from build123d import *

# Parameters (mm, degrees)
F0_R     = 100
F0_R_2   = 9
F0_R_3   = 50
F0_R_4   = 40
F1_DEPTH = 20
F2_DEPTH = 500
F3_R     = 100
F3_R_2   = 9
F3_R_3   = 50
F3_R_4   = 40
F4_DEPTH = 20


with BuildPart() as f1:
    # F0 (on Front) → F1 (new body)
    with BuildSketch(Plane.XZ):
        Circle(F0_R)
        with Locations((-56.5685424949, -56.5685424949)):
            Circle(F0_R_2, mode=Mode.SUBTRACT)
        with Locations((0, -80)):
            Circle(F0_R_2, mode=Mode.SUBTRACT)
        with Locations((56.5685424949, -56.5685424949)):
            Circle(F0_R_2, mode=Mode.SUBTRACT)
        with Locations((-80, 0)):
            Circle(F0_R_2, mode=Mode.SUBTRACT)
        with Locations((-56.5685424949, 56.5685424949)):
            Circle(F0_R_2, mode=Mode.SUBTRACT)
        Circle(F0_R_3, mode=Mode.SUBTRACT)
        with Locations((80, 0)):
            Circle(F0_R_2, mode=Mode.SUBTRACT)
        with Locations((0, 80)):
            Circle(F0_R_2, mode=Mode.SUBTRACT)
        with Locations((56.5685424949, 56.5685424949)):
            Circle(F0_R_2, mode=Mode.SUBTRACT)
        Circle(F0_R_3)
        Circle(F0_R_4, mode=Mode.SUBTRACT)
    extrude(amount=F1_DEPTH)

    # F0 (on Front) → F2 (join)
    with BuildSketch(Plane.XZ):
        Circle(F0_R_3)
        Circle(F0_R_4, mode=Mode.SUBTRACT)
    extrude(amount=F2_DEPTH)

    # F3 (on face) → F4 (join)
    with BuildSketch(Plane.XZ.offset(500)):
        Circle(F3_R)
        with Locations((-56.5685424949, -56.5685424949)):
            Circle(F3_R_2, mode=Mode.SUBTRACT)
        with Locations((0, -80)):
            Circle(F3_R_2, mode=Mode.SUBTRACT)
        with Locations((56.5685424949, -56.5685424949)):
            Circle(F3_R_2, mode=Mode.SUBTRACT)
        with Locations((-80, 0)):
            Circle(F3_R_2, mode=Mode.SUBTRACT)
        with Locations((-56.5685424949, 56.5685424949)):
            Circle(F3_R_2, mode=Mode.SUBTRACT)
        Circle(F3_R_3, mode=Mode.SUBTRACT)
        with Locations((80, 0)):
            Circle(F3_R_2, mode=Mode.SUBTRACT)
        with Locations((0, 80)):
            Circle(F3_R_2, mode=Mode.SUBTRACT)
        with Locations((56.5685424949, 56.5685424949)):
            Circle(F3_R_2, mode=Mode.SUBTRACT)
        Circle(F3_R_3)
        Circle(F3_R_4, mode=Mode.SUBTRACT)
    extrude(amount=F4_DEPTH)


solid = f1.part
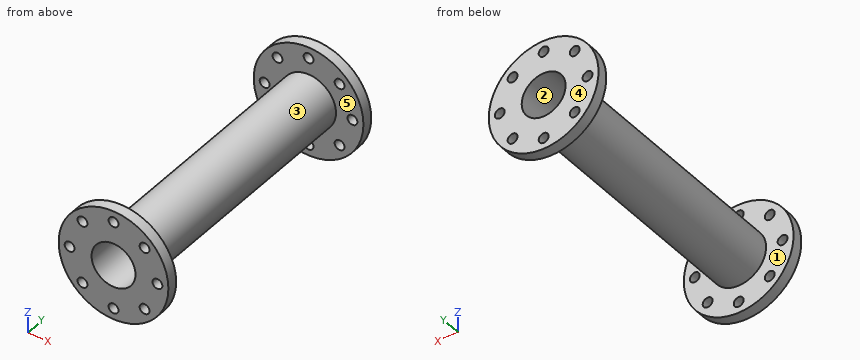
The model under review builds one solid part; all positions refer to its coordinate system, in mm. Face numbers are marked on the shaded views. A direction names the side the tool comes from. Coordinates: 2 decimals unless noted, no trailing zeros. Write each loop counter-clockwise with the first axis right and the second up, starting at its lowest first coordinate (ties: lowest second). Pieces come first, ordered by that corner, then holes. Notation, with made-up numbers: (51.25, 59.25) - (68.25, 59.25) arc R29 cw to (68.25, 91.25) - close; hole circle Ø6 at (2.5, 81). An arc over 180 degrees is marked (long way). Answer as CSV lines item,"result".
(1) Mouldability with a two-part tool opening along X and no side actions: class the marked faces 1, 2 and 3 as pulls with the +X half, pulls with the -X half, needs draft (parallel to the pull), parting line crosses it, or undercut.
Data:
face 1,"needs draft"
face 2,"undercut"
face 3,"parting line crosses it"
(2) For line 1 along Y through (x, z) = (-75, 43); line 2 along Z through (x, y) = (0, -13.5); line 3 along Z through (x, y) = (80, -5.25), list the stretches that pass through material, from the lowest coordinate up. Write a range as [from, to].
Data:
line 1,"y = [-520, -500], [-20, 0]"
line 2,"z = [-100, -89], [-71, -40], [40, 71], [89, 100]"
line 3,"z = [-60, -9], [9, 60]"
(3) We need section B-B (z = -80). Give the boundary of the cut face in (x, y).
Data:
outline,"(-60, -520) - (-9, -520) - (-9, -500) - (-60, -500) - close; (-60, -20) - (-9, -20) - (-9, 0) - (-60, 0) - close; (9, -520) - (60, -520) - (60, -500) - (9, -500) - close; (9, -20) - (60, -20) - (60, 0) - (9, 0) - close"
(4) We need section C-C (x = 0). Count the separate pieces of the cut face and the enclosed holes in it, plus the area to 3 significant figures.
Data:
separate pieces,"6"
enclosed holes,"0"
area,"13,000 mm2"
(5) Clearance check with flat-ended pins moving along their axes: pin 1 Ø14.5 at (x, z) = (80, 0) entering from -Y; pin 2 Ø12 at (y, z) = (-456.5, 35.5) entering from +X; pin 3 Ø2 at (x, y) = (-46.5, -297) entering from -Z; pin 4 Ø4 at (x, y) = (37, -89) entering from -Z. State where each tip first meets the part, or that it passes through.
Data:
pin 1,"passes through"
pin 2,"stops at x = 40.37"
pin 3,"stops at z = -20.73"
pin 4,"stops at z = -35.71"
(6) Tool access review of the marked faces 4 and 5: name each direction out of +Z, -Z, +X, -X, +Y, -Y from which nothing blocks a thin tool from reaching the whole face with its end or side.
Data:
face 4,"+Z, -Z, +X, -X, +Y"
face 5,"none"
(7) We need section A-A (x = -80). Give the boundary of the cut face in (y, z), plus the area to 3 significant figures.
Data:
outline,"(-520, -60) - (-500, -60) - (-500, -9) - (-520, -9) - close; (-520, 9) - (-500, 9) - (-500, 60) - (-520, 60) - close; (-20, -60) - (0, -60) - (0, -9) - (-20, -9) - close; (-20, 9) - (0, 9) - (0, 60) - (-20, 60) - close"
area,"4,080 mm2"
